Model file for the job. Use its own axes, mm. Face numbers are marked on the shaded views. A direction names the side the tool comes from. Give positions to 0.01 mm unless a question says otherwise; leave off trailing zeros. Order: outer loops, then holes, each group sorted by start corner. A loop starts at its lowest first (then second) coordinate and runs counter-clockwise, first axis right, second up. Notation, with made-up numbers: (-19, 25.25) -> (16, 25.25) arc R9 ccw to (16, 35.25) -> close; hole circle Ø2 at (12.5, 46). An arc over 180 degrees is marked (long way). Answer in a Markdown table with one row per item. Add a question column.
from build123d import *

# Parameters (mm, degrees)
SKETCH1_W           = 30
SKETCH1_H           = 30
BOSS_EXTRUDE1_DEPTH = 5
SKETCH2_R           = 9
BOSS_EXTRUDE2_DEPTH = 5.8
BOSS_EXTRUDE2_TAPER = 35
SKETCH4_R           = 5
CUT_EXTRUDE2_DEPTH  = 8
BOSS_EXTRUDE3_DEPTH = 7.5
CHAMFER1_SIZE       = 1
FILLET2_R           = 4
SKETCH6_W           = 30
SKETCH6_H           = 2
CUT_EXTRUDE3_DEPTH  = 36.210220534
CHAMFER2_SIZE       = 0.6


with BuildPart() as part:
    # Sketch1 → Boss-Extrude1 (new body)
    with BuildSketch(Plane(origin=(0, 0, 0), x_dir=(1, 0, 0), z_dir=(0, 1, 0))):
        Rectangle(SKETCH1_W, SKETCH1_H)
    extrude(amount=BOSS_EXTRUDE1_DEPTH)

    # Sketch2 → Boss-Extrude2 (add)
    with BuildSketch(Plane(origin=(0, 5, 0), x_dir=(1, 0, 0), z_dir=(0, 1, 0))):
        Circle(SKETCH2_R)
    extrude(amount=BOSS_EXTRUDE2_DEPTH, taper=BOSS_EXTRUDE2_TAPER)

    # Sketch4 → Cut-Extrude2 (cut)
    with BuildSketch(Plane(origin=(0, 10.8, 0), x_dir=(1, 0, 0), z_dir=(0, 1, 0))):
        with Locations(Location((0, 0, 0), (0, 0, 270))):
            Circle(SKETCH4_R)
    extrude(amount=-CUT_EXTRUDE2_DEPTH, mode=Mode.SUBTRACT)

    # Sketch5 → Boss-Extrude3 (add)
    with BuildSketch(Plane(origin=(0, 2.8, 0), x_dir=(1, 0, 0), z_dir=(0, 1, 0))):
        with BuildLine():
            Line((-1.533599577, 4.863956449), (-0.917152688, 2.9088367))
            ThreePointArc((-0.917152688, 2.9088367), (0, 3.05), (0.917152688, 2.9088367))
            Line((0.917152688, 2.9088367), (1.533599577, 4.863956449))
            ThreePointArc((1.533599577, 4.863956449), (0, 5.1), (-1.533599577, 4.863956449))
        make_face()
        with BuildLine():
            Line((3.445510059, -3.760114418), (2.060550133, -2.248695877))
            ThreePointArc((2.060550133, -2.248695877), (2.641377482, -1.525), (2.977702822, -0.660140823))
            Line((2.977702822, -0.660140823), (4.979109636, -1.103842031))
            ThreePointArc((4.979109636, -1.103842031), (4.416729559, -2.55), (3.445510059, -3.760114418))
        make_face()
        with BuildLine():
            Line((-4.979109636, -1.103842031), (-2.977702822, -0.660140823))
            ThreePointArc((-2.977702822, -0.660140823), (-2.641377482, -1.525), (-2.060550133, -2.248695877))
            Line((-2.060550133, -2.248695877), (-3.445510059, -3.760114418))
            ThreePointArc((-3.445510059, -3.760114418), (-4.416729559, -2.55), (-4.979109636, -1.103842031))
        make_face()
    extrude(amount=BOSS_EXTRUDE3_DEPTH)

    # Chamfer1
    chamfer1_edges = [part.edges().sort_by_distance(p)[0] for p in [
        (0, 0, 15),
        (-15, 0, 0),
        (0, 0, -15),
        (15, 0, 0),
        (15, 2.5, 15),
        (-15, 2.5, 15),
        (-15, 2.5, -15),
        (15, 2.5, -15),
    ]]
    chamfer(chamfer1_edges, length=CHAMFER1_SIZE)

    # Fillet2
    fillet2_edges = [part.edges().sort_by_distance(p)[0] for p in [
        (-9, 5, 0),
    ]]
    fillet(fillet2_edges, radius=FILLET2_R)

    # Sketch6 → Cut-Extrude3 (cut, through all)
    with BuildSketch(Plane.XY.offset(15)):
        with Locations((0, 11)):
            Rectangle(SKETCH6_W, SKETCH6_H)
    extrude(amount=-CUT_EXTRUDE3_DEPTH, mode=Mode.SUBTRACT)

    # Chamfer2
    chamfer2_edges = [part.edges().sort_by_distance(p)[0] for p in [
        (-4.330127019, 2.8, -2.5),
        (-1.210340843, 2.8, -3.838710727),
        (1.210340843, 2.8, -3.838710727),
        (0, 2.8, -3.05),
        (4.330127019, 2.8, -2.5),
        (3.929591429, 2.8, 0.871169446),
        (2.719250586, 2.8, 2.967541281),
        (2.641377482, 2.8, 1.525),
        (0, 2.8, 5),
        (-2.719250586, 2.8, 2.967541281),
        (-3.929591429, 2.8, 0.871169446),
        (-2.641377482, 2.8, 1.525),
    ]]
    chamfer(chamfer2_edges, length=CHAMFER2_SIZE)


solid = part.part
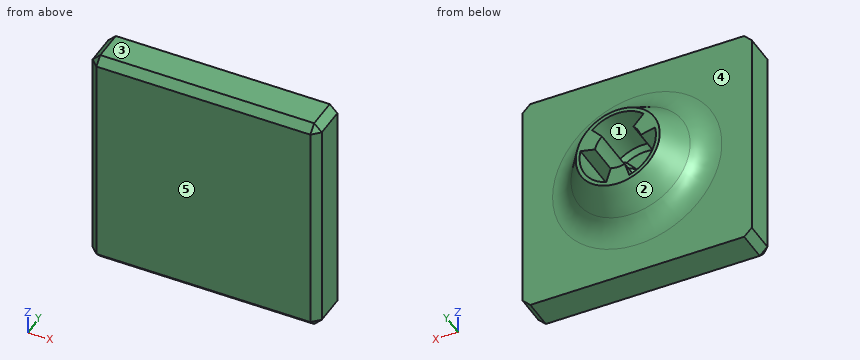
Item 1: Saw through at B-B on y = 8. List the corners of the cut face in (x, z).
Item 2: Which spindle directions (+Z, -Z, +X, -X, +Y, -Y) get a long thin tool onto all of the face, cutting with end or side? Do the marked faces 4 and 5. Say none if no direction does.
Item 3: Two-plate mould, pull along X, no slides. Class the marked faces 1, 2 and 3: pulls with the +X half, pulls with the -X half, needs draft (parallel to the pull), parting line crosses it, or undercut.
Item 4: Saw through at C-C on x = 0. List the corners of the cut face in (y, z).
Item 5: Saw through at A-A on z = 13.25. List the corners of the cut face in (x, y).
Item 6: Wall check: line 1 (Y direction, x = 0.25, z = 12.25); line 2 (Z direction, x = -2, y = 4.75); line 3 (X direction, y = 5.5, z = 2.5). Give the ranges that are in metal, low to high.
Item 7: Pin check, flat tips, straight feed: pin 1 Ø5 at (y, z) = (9, -8) entering from -X; pin 2 Ø12 at (x, z) = (9, -11) entering from +Y; pin 3 Ø4 at (x, y) = (5.5, 8.5) entering from -Z. Stop position of each tip, or through.
Evaluation:
| question | item | result |
|---|---|---|
| 1 | outline | circle Ø13.8 at (0, 0); hole (-4.88, 1.08) arc R5 ccw to (-1.5, -4.77) -> (-0.92, -2.91) arc R3.05 ccw to (0.92, -2.91) -> (1.5, -4.77) arc R5 ccw to (4.88, 1.08) -> (2.98, 0.66) arc R3.05 ccw to (2.06, 2.25) -> (3.38, 3.69) arc R5 ccw to (-3.38, 3.69) -> (-2.06, 2.25) arc R3.05 ccw to (-2.98, 0.66) -> close |
| 2 | face 4 | +Y |
| 2 | face 5 | +Z, -Z, +X, -X, -Y |
| 3 | face 1 | undercut |
| 3 | face 2 | parting line crosses it |
| 3 | face 3 | needs draft |
| 4 | outline | (0, -14) -> (1, -15) -> (5, -15) -> (5, -11.08) arc R4 cw to (6.71, -7.81) -> (10, -5.5) -> (10, -3.05) -> (3.4, -3.05) -> (2.8, -2.45) -> (2.8, 4.4) -> (3.4, 5) -> (10, 5) -> (10, 5.5) -> (6.71, 7.81) arc R4 cw to (5, 11.08) -> (5, 15) -> (1, 15) -> (0, 14) -> close |
| 5 | outline | (-15, 1) -> (-14, 0) -> (14, 0) -> (15, 1) -> (15, 5) -> (-15, 5) -> close |
| 6 | line 1 | y = 0 to 5 |
| 6 | line 2 | z = -15 to -4.58, 4.58 to 15 |
| 6 | line 3 | x = -8.8 to -2.29, 2.29 to 8.8 |
| 7 | pin 1 | stops at x = -4.08 |
| 7 | pin 2 | stops at y = 6.21 |
| 7 | pin 3 | stops at z = -6.35 |
